Geometry check sheet. Reference: drawing and pictorial views, mm from the part's lowest x, y, z. A direction names the side the tool comes from. Give positions to 0.01 mm unless a question says otherwise; leave off trailing zeros. Loops run counter-clockwise (first coordinate to the right, second up) from the corner with the lowest first, then second, coordinate; pieces in that order, holes last. Notation, with made-up numbers: (37, 70.25) - (93, 70.25) arc R27 ccw to (93, 87.25) - close; hole circle Ø10 at (53.5, 16). An arc over 180 degrees is marked (long way). One line per question, with ' | ' between items. Start each with the question number.
1. Depth check by flat-ended pin: pin 1 Ø3 at (x, z) = (25.5, 71) entering from -Y. Enter the tip coordinate at first touch or a pass-through.
2. Section check C-C, the plane x = 44.5. Enter the section's corners in (y, z).
3. Thickness scan on line 1 along X through (y, z) = (13, 12); line 2 along Z through (x, y) = (20, 12); line 3 along Y through (x, z) = (48, 38.5). Record the ranges inside material, lowest first. Write a range as from..to.
4. Tool access check on the marked faces 5 and 6. Record the directions out of +Z, -Z, +X, -X, +Y, -Y that give a thin tool (end or side, any length) a straight path to the whole face; none if there is none.
5. Section check A-A, the plane y = 6. Enter the section's corners in (x, z).
6. Section check B-B, the plane z = 9. Enter the section's corners in (x, y).
7. Mould release check, pull along X, two halves, no side actions. Record for the marked faces 1, 2, 3 and 4: +X half, -X half, draft (parallel to the pull), parting line (faces both ways), or undercut.
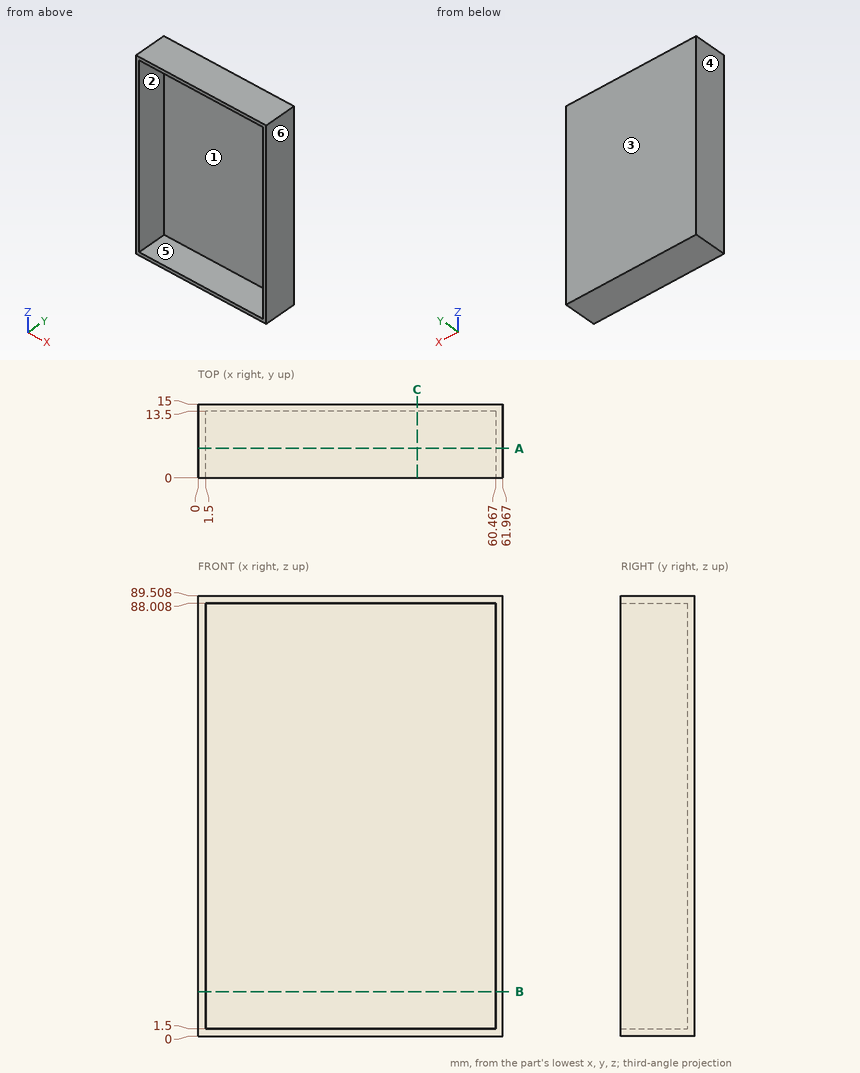
Results list:
1) pin 1: y = 13.5
2) outline: (0, 0) - (15, 0) - (15, 89.51) - (0, 89.51) - (0, 88.01) - (13.5, 88.01) - (13.5, 1.5) - (0, 1.5) - close
3) line 1: 0..1.5, 60.47..61.97 | line 2: 0..1.5, 88.01..89.51 | line 3: 13.5..15
4) face 5: -Y | face 6: +Z, -Z, +X, +Y, -Y
5) outline: (0, 0) - (61.97, 0) - (61.97, 89.51) - (0, 89.51) - close; hole (1.5, 1.5) - (60.47, 1.5) - (60.47, 88.01) - (1.5, 88.01) - close
6) outline: (0, 0) - (1.5, 0) - (1.5, 13.5) - (60.47, 13.5) - (60.47, 0) - (61.97, 0) - (61.97, 15) - (0, 15) - close
7) face 1: undercut | face 2: undercut | face 3: draft | face 4: -X half
